Check sheet for the modelled part. Datum: model origin and axes. Units: mm. A direction names the side the tool comes from. Coordinates: 2 decimals unless noted, no trailing zeros. Order: outer loops, then holes, each group sorted by start corner. A loop starts at its lowest first (then second) coordinate and runs counter-clockwise, first axis right, second up.
1. Draft check along X on faces 1 (the flat face through (-55, -5, 0)), 2 (the cylindrical face through (-30, -5, -15)), 3 (the flat face through (25, -25, 1)). Enter one of: released by +X, released by -X, zero draft, split by the parting line, or undercut.
2. Cross-section at B-B (y = -8.5). Enter the section's corners in (x, z).
3. Cross-section at C-C (x = -30). Enter the section's corners in (y, z).
4. Thickness scan on line 1 (Y direction, x = 1, z = -35.5); line 2 (Y direction, x = 19.5, z = -26.5); line 3 (X direction, y = -7.5, z = -3). Record the ranges inside material, lowest first.
5. Cross-section at A-A (z = -9). Enter the section's corners in (x, y), then the cut area to 3 significant figures.
6. Gauge pin test, flat ends, axial feed: pin 1 Ø2 at (x, z) = (-2.5, 15.5) entering from -Y; pin 2 Ø6 at (x, y) = (32, -5) entering from -Z; pin 3 Ø1 at (y, z) = (-17, -19.5) entering from +X; pin 4 Ø3 at (x, z) = (-8.5, 23) entering from +Y. Record the tip position at first contact, or that the pin passes through.
7. Set-up check for faces 4 (the flat face through (9, -20, 1)), 5 (the flat face through (40, -30, 1)): record each of +Z, -Z, +X, -X, +Y, -Y from which the full face is reachable in a straight line by a thin tool's end or side.
8. Cross-section at D-D (z = 10.5). Enter the section's corners in (x, y), then the cut area to 3 significant figures.
```python
from build123d import *

# Parameters (mm, degrees)
F1_DEPTH = 30
F2_DEPTH = 20
F3_DEPTH = 10


with BuildPart() as f1:
    # F0 (on Front) → F1 (new body)
    with BuildSketch(Plane.XZ):
        with BuildLine():
            ThreePointArc((50, 0), (42.67767, 17.67767), (25, 25))
            Line((25, 25), (25, 0))
            Line((25, 0), (25, -25))
            ThreePointArc((25, -25), (42.67767, -17.67767), (50, 0))
        make_face()
        with BuildLine():
            ThreePointArc((25, -40), (53.284271, -28.284271), (65, 0))
            ThreePointArc((65, 0), (53.284271, 28.284271), (25, 40))
            Line((25, 40), (25, 25))
            ThreePointArc((25, 25), (42.67767, 17.67767), (50, 0))
            ThreePointArc((50, 0), (42.67767, -17.67767), (25, -25))
            Line((25, -25), (25, -40))
        make_face()
    extrude(amount=F1_DEPTH)

    # F0 (on Front) → F2 (join)
    with BuildSketch(Plane.XZ):
        with BuildLine():
            ThreePointArc((25, 40), (-3.284271, 28.284271), (-15, 0))
            ThreePointArc((-15, 0), (-3.284271, -28.284271), (25, -40))
            Line((25, -40), (25, -25))
            ThreePointArc((25, -25), (0, 0), (25, 25))
            Line((25, 25), (25, 40))
        make_face()
        with BuildLine():
            Line((25, 0), (25, 25))
            ThreePointArc((25, 25), (0, 0), (25, -25))
            Line((25, -25), (25, 0))
        make_face()
    extrude(amount=F2_DEPTH)

    # F0 (on Front) → F3 (join)
    with BuildSketch(Plane.XZ):
        with BuildLine():
            Line((-45, 0), (-65, 0))
            ThreePointArc((-65, 0), (0, -65), (65, 0))
            ThreePointArc((65, 0), (53.284271, -28.284271), (25, -40))
            ThreePointArc((25, -40), (-3.284271, -28.284271), (-15, 0))
            ThreePointArc((-15, 0), (-30, -15), (-45, 0))
        make_face()
    extrude(amount=F3_DEPTH)


solid = f1.part
```
Data:
1. face 1: zero draft
1. face 2: undercut
1. face 3: released by -X
2. outline: (-65, 0) arc R65 ccw to (65, 0) arc R40 ccw to (25, 40) arc R40 ccw to (-15, 0) arc R15 cw to (-45, 0) - close
3. outline: (-10, -57.66) - (0, -57.66) - (0, -15) - (-10, -15) - close
4. line 1: y = -10 to 0
4. line 2: y = -20 to 0
4. line 3: x = -64.93 to -44.7, -15.3 to 64.93
5. outline: (-64.37, -10) - (-42, -10) - (-42, 0) - (-64.37, 0) - close; (-18, -10) - (-13.97, -10) - (-13.97, -20) - (25, -20) - (25, -30) - (63.97, -30) - (63.97, -10) - (64.37, -10) - (64.37, 0) - (-18, 0) - close
5. area: 2,220 mm2
6. pin 1: stops at y = -20
6. pin 2: stops at z = -58.17
6. pin 3: stops at x = 60.2
6. pin 4: stops at y = 0
7. face 4: +Z, -Z, -X, -Y
7. face 5: +Z, -Z, +X, -X, -Y
8. outline: (-13.6, -20) - (25, -20) - (25, -30) - (63.6, -30) - (63.6, 0) - (-13.6, 0) - close
8. area: 1,930 mm2
